from build123d import *

# Parameters (mm, degrees)
BOSS_EXTRUDE1_DEPTH = 31.75
SKETCH3_R           = 2.4892
CUT_EXTRUDE1_DEPTH  = 65.185965172


with BuildPart() as part:
    # Sketch1 → Boss-Extrude1 (new, symmetric)
    with BuildSketch(Plane.XY):
        with BuildLine():
            Line((-0.893039494, 6.816751826), (-5.456960506, 4.181770802))
            ThreePointArc((-5.456960506, 4.181770802), (-5.953924651, 3.4375), (-6.35, 2.634981025))
            Line((-6.35, 2.634981025), (-6.35, -2.634981025))
            ThreePointArc((-6.35, -2.634981025), (-5.953924651, -3.4375), (-5.456960506, -4.181770802))
            Line((-5.456960506, -4.181770802), (-0.893039494, -6.816751826))
            ThreePointArc((-0.893039494, -6.816751826), (0, -6.875), (0.893039494, -6.816751826))
            Line((0.893039494, -6.816751826), (5.456960506, -4.181770802))
            ThreePointArc((5.456960506, -4.181770802), (5.953924651, -3.4375), (6.35, -2.634981025))
            Line((6.35, -2.634981025), (6.35, 2.634981025))
            ThreePointArc((6.35, 2.634981025), (5.953924651, 3.4375), (5.456960506, 4.181770802))
            Line((5.456960506, 4.181770802), (0.893039494, 6.816751826))
            ThreePointArc((0.893039494, 6.816751826), (0, 6.875), (-0.893039494, 6.816751826))
        make_face()
    extrude(amount=BOSS_EXTRUDE1_DEPTH, both=True)

    # Sketch3 → Cut-Extrude1 (cut, through all)
    with BuildSketch(Plane.XY.offset(31.75)):
        Circle(SKETCH3_R)
    extrude(amount=-CUT_EXTRUDE1_DEPTH, mode=Mode.SUBTRACT)


solid = part.part
Source: CAD feature listing. Evaluate the final solid. Frame: model axes, mm. Coordinates: 2 decimals unless noted, no trailing zeros. Loops run counter-clockwise (first coordinate to the right, second up) from the corner with the lowest first, then second, coordinate; pieces in that order, holes last. Notation, with made-up numbers: (89.5, 3.5) - (138.5, 3.5) arc R10 cw to (138.5, 22.5) - close; hole circle Ø11 at (0.25, -36.5). An arc over 180 degrees is marked (long way). Return JSON: item names as keys, results as strings.
Q1. Material intervals for line 1 along Y through (x, z) = (0, 0.5) (3 decimals); line 2 along X through (y, z) = (2, 3.5); line 3 along X through (y, z) = (-1.75, -12), sorted ascending.
Results:
{"line 1": "-6.875 to -2.489, 2.489 to 6.875", "line 2": "-6.35 to -1.48, 1.48 to 6.35", "line 3": "-6.35 to -1.77, 1.77 to 6.35"}
Q2. Section A-A, the plane y = 0. Return loops of the section in (x, z).
Results:
{"outline": "(-6.35, -31.75) - (-2.49, -31.75) - (-2.49, 31.75) - (-6.35, 31.75) - close; (2.49, -31.75) - (6.35, -31.75) - (6.35, 31.75) - (2.49, 31.75) - close"}
Q3. Contact query for flat-ended pins moving along their axis: P1, Ø1, axis at x = -2.5, z = 0, coming from the -Y side; P2, Ø5, axis at x = 0, y = 1.5, coming from the +Z side; P3, Ø5, axis at x = -4, z = -10, coming from the -Y side. Output: stop coordinate, or through.
Results:
{"P1": "y = -6.18", "P2": "z = 31.75", "P3": "y = -6.47"}
Q4. Mould query, pull axis X, two halves, no side actions, for faces 1 (the flat face through (-6.35, 0, 0)), 2 (the flat face through (6.35, 0, 0)), 3 (the cylindrical face through (2.374, 0.748, 0.444)), 4 (the flat face through (3, 0, -31.75)). Classes: released by +X, released by -X, zero draft, split by the parting line, or undercut.
Results:
{"face 1": "released by -X", "face 2": "released by +X", "face 3": "undercut", "face 4": "zero draft"}
Q5. Section B-B, the plane z = -11. Return loops of the section in (x, y) (3 decimals), plus the area to 3 significant figures.
Results:
{"outline": "(-6.35, -2.635) arc R6.875 ccw to (-5.457, -4.182) - (-0.893, -6.817) arc R6.875 ccw to (0.893, -6.817) - (5.457, -4.182) arc R6.875 ccw to (6.35, -2.635) - (6.35, 2.635) arc R6.875 ccw to (5.457, 4.182) - (0.893, 6.817) arc R6.875 ccw to (-0.893, 6.817) - (-5.457, 4.182) arc R6.875 ccw to (-6.35, 2.635) - close; hole circle Ø4.978 at (0, 0)", "area": "118 mm2"}
Q6. Section D-D, the plane y = 3.5. Return loops of the section in (x, z), plus the area to 3 significant figures.
Results:
{"outline": "(-5.92, -31.75) - (5.92, -31.75) - (5.92, 31.75) - (-5.92, 31.75) - close", "area": "752 mm2"}
Q7. Section C-C, the plane x = 0. Return loops of the section in (y, z) (3 decimals), plus the area to 3 significant figures.
Results:
{"outline": "(-6.875, -31.75) - (-2.489, -31.75) - (-2.489, 31.75) - (-6.875, 31.75) - close; (2.489, -31.75) - (6.875, -31.75) - (6.875, 31.75) - (2.489, 31.75) - close", "area": "557 mm2"}
